The listing builds one solid part. Answer for the finished solid, in the listing's coordinates (mm). Give positions to 0.01 mm unless a question says otherwise; leave off trailing zeros. Loops run counter-clockwise (first coordinate to the right, second up) from the corner with the lowest first, then second, coordinate; pieces in that order, holes last.
Item 1: Section B-B, the plane z = -68 is taken. Give the vertices of the cut face in (x, y).
Item 2: Each of these flat-tipped pins is pushed along its axis until it touches: pin 1 Ø1.5 at (x, y) = (329, 1.5) entering from +Z; pin 2 Ø1.5 at (y, z) = (1, -54.5) entering from +X; pin 3 Ø0.9 at (x, y) = (328, 2) entering from -Z. Where does it stop, or does it pass through?
Item 3: The mould has two halves that part along Z. Classify faces 1 (the face through (18.828, 1.479, -188.923)), 2 (the face through (4.51, 1.52, -4.28)), 3 (the face through (325.49, 1.52, -205.72)), 4 (the face through (163, 0, -106)): pulls with the +Z half, pulls with the -Z half, needs draft (parallel to the pull), parting line crosses it, or undercut.
Item 4: Section D-D, the plane y = 0.8 is taken. Give the number of separate pieces and of enclosed holes in the cut face, and give its area (3 significant figures).
Item 5: Consider line 1 along X through (y, z) = (1.6, -99); line 2 along X through (y, z) = (0.8, -180); line 3 along X through (y, z) = (1.4, -78). Determine where each line is inside the solid, lowest interval first.
Item 6: Section C-C, the plane x = 20 is taken. Give the vertices of the cut face in (y, z).
Item 7: Section A-A, the plane z = -180 is taken. Give the vertices of the cut face in (x, y), and give its area (3 significant figures).
from build123d import *

# Parameters (mm, degrees)
ESQUISSE1_R      = 2.5
ESQUISSE1_R_2    = 9
EXTRUSION1_DEPTH = 3
CONG_1_R         = 15
EXTRUSION2_REACH = 5
ESQUISSE2_W      = 300
ESQUISSE2_H      = 3
ESQUISSE2_W_2    = 3
ESQUISSE2_H_2    = 91
ESQUISSE2_H_3    = 79
EXTRUSION3_REACH = 5
ESQUISSE3_W      = 230
ESQUISSE3_H      = 60


with BuildPart() as part:
    # Esquisse1 → Extrusion1 (new body)
    with BuildSketch(Plane(origin=(0, 0, 0), x_dir=(1, 0, 0), z_dir=(0, 1, 0))):
        Polygon((0, 0), (24, 0), (24, 100), (165, 100), (306, 100), (306, 0), (330, 0), (330, 210), (0, 210), align=None)
        with Locations((10, 200)):
            Circle(ESQUISSE1_R, mode=Mode.SUBTRACT)
        with Locations((320, 200)):
            Circle(ESQUISSE1_R, mode=Mode.SUBTRACT)
        with Locations((10, 99)):
            Circle(ESQUISSE1_R, mode=Mode.SUBTRACT)
        with Locations((320, 99)):
            Circle(ESQUISSE1_R, mode=Mode.SUBTRACT)
        with Locations((10, 10)):
            Circle(ESQUISSE1_R, mode=Mode.SUBTRACT)
        with Locations((320, 10)):
            Circle(ESQUISSE1_R, mode=Mode.SUBTRACT)
        with Locations((20, 180)):
            Circle(ESQUISSE1_R_2, mode=Mode.SUBTRACT)
    extrude(amount=EXTRUSION1_DEPTH)

    # Congé1
    cong_1_edges = [part.edges().sort_by_distance(p)[0] for p in [
        (0, 1.5, -210),
        (330, 1.5, -210),
        (330, 1.5, 0),
        (0, 1.5, 0),
    ]]
    fillet(cong_1_edges, radius=CONG_1_R)

    # Esquisse2 → Extrusion2 (cut, up to next)
    with BuildSketch(Plane(origin=(0, 3, 0), x_dir=(1, 0, 0), z_dir=(0, 1, 0)), mode=Mode.PRIVATE) as extrusion2_sk1:
        with Locations((165, 208.5)):
            Rectangle(ESQUISSE2_W, ESQUISSE2_H)
    extrusion2_tool1 = extrude(extrusion2_sk1.sketch, amount=-EXTRUSION2_REACH, mode=Mode.PRIVATE) & part.part
    add(extrusion2_tool1.solids().sort_by_distance((165, 3, -208.5))[0], mode=Mode.SUBTRACT)
    # Esquisse2 → Extrusion2 (cut, up to next)
    with BuildSketch(Plane(origin=(0, 3, 0), x_dir=(1, 0, 0), z_dir=(0, 1, 0)), mode=Mode.PRIVATE) as extrusion2_sk2:
        with Locations((1.5, 149.5)):
            Rectangle(ESQUISSE2_W_2, ESQUISSE2_H_2)
    extrusion2_tool2 = extrude(extrusion2_sk2.sketch, amount=-EXTRUSION2_REACH, mode=Mode.PRIVATE) & part.part
    add(extrusion2_tool2.solids().sort_by_distance((1.5, 3, -149.5))[0], mode=Mode.SUBTRACT)
    # Esquisse2 → Extrusion2 (cut, up to next)
    with BuildSketch(Plane(origin=(0, 3, 0), x_dir=(1, 0, 0), z_dir=(0, 1, 0)), mode=Mode.PRIVATE) as extrusion2_sk3:
        with Locations((1.5, 54.5)):
            Rectangle(ESQUISSE2_W_2, ESQUISSE2_H_3)
    extrusion2_tool3 = extrude(extrusion2_sk3.sketch, amount=-EXTRUSION2_REACH, mode=Mode.PRIVATE) & part.part
    add(extrusion2_tool3.solids().sort_by_distance((1.5, 3, -54.5))[0], mode=Mode.SUBTRACT)
    # Esquisse2 → Extrusion2 (cut, up to next)
    with BuildSketch(Plane(origin=(0, 3, 0), x_dir=(1, 0, 0), z_dir=(0, 1, 0)), mode=Mode.PRIVATE) as extrusion2_sk4:
        with Locations((328.5, 54.5)):
            Rectangle(ESQUISSE2_W_2, ESQUISSE2_H_3)
    extrusion2_tool4 = extrude(extrusion2_sk4.sketch, amount=-EXTRUSION2_REACH, mode=Mode.PRIVATE) & part.part
    add(extrusion2_tool4.solids().sort_by_distance((328.5, 3, -54.5))[0], mode=Mode.SUBTRACT)
    # Esquisse2 → Extrusion2 (cut, up to next)
    with BuildSketch(Plane(origin=(0, 3, 0), x_dir=(1, 0, 0), z_dir=(0, 1, 0)), mode=Mode.PRIVATE) as extrusion2_sk5:
        with Locations((328.5, 149.5)):
            Rectangle(ESQUISSE2_W_2, ESQUISSE2_H_2)
    extrusion2_tool5 = extrude(extrusion2_sk5.sketch, amount=-EXTRUSION2_REACH, mode=Mode.PRIVATE) & part.part
    add(extrusion2_tool5.solids().sort_by_distance((328.5, 3, -149.5))[0], mode=Mode.SUBTRACT)

    # Esquisse3 → Extrusion3 (cut, up to next)
    with BuildSketch(Plane(origin=(0, 3, 0), x_dir=(1, 0, 0), z_dir=(0, 1, 0)), mode=Mode.PRIVATE) as extrusion3_sk1:
        with Locations((165, 177)):
            Rectangle(ESQUISSE3_W, ESQUISSE3_H)
    extrusion3_tool1 = extrude(extrusion3_sk1.sketch, amount=-EXTRUSION3_REACH, mode=Mode.PRIVATE) & part.part
    add(extrusion3_tool1.solids().sort_by_distance((165, 3, -177))[0], mode=Mode.SUBTRACT)


solid = part.part
Worked answers:
1. outline: (3, 0) - (24, 0) - (24, 3) - (3, 3) - close; (306, 0) - (327, 0) - (327, 3) - (306, 3) - close
2. pin 1: stops at z = -7.97
2. pin 2: stops at x = 327
2. pin 3: stops at z = -203.22
3. face 1: undercut
3. face 2: pulls with the +Z half
3. face 3: pulls with the -Z half
3. face 4: needs draft
4. separate pieces: 1
4. enclosed holes: 7
4. area: 24,800 mm2
5. line 1: x = 0 to 7.5, 12.5 to 24, 306 to 317.5, 322.5 to 330
5. line 2: x = 3 to 11, 29 to 50, 280 to 327
5. line 3: x = 3 to 24, 306 to 327
6. outline: (0, -207) - (3, -207) - (3, -189) - (0, -189) - close; (0, -171) - (3, -171) - (3, 0) - (0, 0) - close
7. outline: (3, 0) - (11, 0) - (11, 3) - (3, 3) - close; (29, 0) - (50, 0) - (50, 3) - (29, 3) - close; (280, 0) - (327, 0) - (327, 3) - (280, 3) - close
7. area: 228 mm2
